```python
from build123d import *

# Parameters (mm, degrees)
BRIDA_BASE1_DEPTH            = 1.5875
TALADRO_DE_MARGEN_PARA_M61_D = 6.6
CROQUIS7_W                   = 314.97561102
CROQUIS7_H                   = 1242.8481637
CORTAR_EXTRUIR2_DEPTH        = 3200


# Sheet-metal steps are written as plain solids
with BuildPart() as part:
    # Croquis1 → Brida base1 (new body)
    with BuildSketch(Plane.XY):
        Polygon((-251.585, -706), (251.585, -1050.4), (251.585, -706), (251.585, 706), (251.585, 1050.4), (-251.585, 706), align=None)
    extrude(amount=-BRIDA_BASE1_DEPTH)

    # Taladro de margen para M61 (through all)
    with Locations(Plane.XY):
        with Locations((-231.585, 695.452987896), (-157.316935544, 746.288552238), (-83.048871087, 797.124116579), (-8.780806631, 847.95968092), (65.487257826, 898.795245261), (139.755322282, 949.630809603), (214.023386739, 1000.466373944), (65.487257826, -898.795245261), (-8.780806631, -847.95968092), (-83.048871087, -797.124116579), (-157.316935544, -746.288552238), (-231.585, -695.452987896), (214.023386739, -1000.466373944), (139.755322282, -949.630809603), (-231.585, -521.452987896), (-231.585, -347.452987896), (-231.585, -173.452987896), (-231.585, 0.547012104), (-231.585, 174.547012104), (-231.585, 348.547012104), (-231.585, 522.547012104), (231.585, 522.547012104), (231.585, 348.547012104), (231.585, 174.547012104), (231.585, 0.547012104), (231.585, -173.452987896), (231.585, -347.452987896), (231.585, -521.452987896), (231.585, -695.452987896), (231.585, -869.452987896), (231.585, 696.547012104), (231.585, 870.547012104)):
            Hole(TALADRO_DE_MARGEN_PARA_M61_D / 2)

    # Croquis7 → Cortar-Extruir2 (cut)
    with BuildSketch(Plane.XY.offset(-1.5875)):
        Rectangle(CROQUIS7_W, CROQUIS7_H)
    extrude(amount=CORTAR_EXTRUIR2_DEPTH, mode=Mode.SUBTRACT)


solid = part.part
```
Here's how the part is built. I have some questions about the finished solid (model axes, mm). Give positions to 0.01 mm unless a question says otherwise; leave off trailing zeros. Order: outer loops, then holes, each group sorted by start corner. A loop starts at its lowest first (then second) coordinate and runs counter-clockwise, first axis right, second up. Notation, with made-up numbers: (10.25, 65.25) - (23.25, 65.25) arc R19 cw to (23.25, 94.25) - close; hole circle Ø9 at (-20, -10). An arc over 180 degrees is marked (long way). Answer as a JSON object with one key per item and string values. Group by question number.
Item 1: If we section it at A-A on x = -113: Please give me the cut outline in (y, z), and give its area (3 significant figures).
Item 2: Please list where these lines run through material, in increasing order: probe 1 along X at (y, z) = (236, -0.5) (3 decimals); probe 2 along Y at (x, z) = (215.5, -1.25); probe 3 along Y at (x, z) = (109, -0.55).
Item 3: If we section it at B-B on y = -40: Please give me the cut outline in (x, z) (1 decimal).
Item 4: For P1, Ø0.5, axis at x = -9.5, z = -0.5, coming from the -Y side, with a flat end and sliding along its axis, tell me the tip position at first contact or that it passes through.
Item 5: If we section it at D-D on x = -193.5: Please give me the cut outline in (y, z).
Item 6: If we section it at C-C on z = -1.2: Give the number of separate pieces and of enclosed holes in the cut face, and give its area (3 significant figures).
Result set:
{
 "1": {"outline": "(-800.86, -1.59) - (-621.42, -1.59) - (-621.42, 0) - (-800.86, 0) - close; (621.42, -1.59) - (800.86, -1.59) - (800.86, 0) - (621.42, 0) - close", "area": "570 mm²"},
 "2": {"probe 1": "-251.585 to -157.488, 157.488 to 251.585", "probe 2": "-1025.7 to -1003.42, -997.52 to 997.52, 1003.42 to 1025.7", "probe 3": "-952.81 to -621.42, 621.42 to 952.81"},
 "3": {"outline": "(-251.6, -1.6) - (-157.5, -1.6) - (-157.5, 0) - (-251.6, 0) - close; (157.5, -1.6) - (251.6, -1.6) - (251.6, 0) - (157.5, 0) - close"},
 "4": {"P1": "y = -871.87"},
 "5": {"outline": "(-745.76, -1.59) - (745.76, -1.59) - (745.76, 0) - (-745.76, 0) - close"},
 "6": {"separate pieces": "1", "enclosed holes": "33", "area": "491,000 mm²"}
}
